Autodesk Inventor part; units mm, degrees
ref_plane "YZ Plane" through (0, 0, 0) normal (1, 0, 0) x (0, 1, 0)
ref_plane "XZ Plane" through (0, 0, 0) normal (0, 1, 0) x (-1, 0, 0)
ref_plane "XY Plane" through (0, 0, 0) normal (0, 0, 1) x (1, 0, 0)
sketch "Szkic1" plane through (0, 0, 0) normal (0, 0, 1) x (1, 0, 0)
  line L0 (6.7664, -3.387) -> (-9.1111, -1.9923)
  arc A0 (6.7664, 3.387) -> (6.7664, -3.387) centre (7.0639, 0) ccw construction
  line L1 (6.7664, 3.387) -> (-9.1111, 1.9923)
  arc A1 (-9.1111, 1.9923) -> (-9.1111, -1.9923) centre (-8.9361, 0) ccw
  circle A2 centre (-5.2361, 0) radius 0.5
  circle A3 centre (-7.1361, 0) radius 0.5
  circle A4 centre (-9.0361, 0) radius 0.5
  circle A5 centre (2.3639, 0) radius 0.5
  circle A6 centre (0.4639, 0) radius 0.5
  circle A7 centre (-1.4361, 0) radius 0.5
  circle A8 centre (-3.3361, 0) radius 0.5
  circle A9 centre (7.0639, 0) radius 3.4 construction
  arc A10 (6.6789, -4.3831) -> (6.6789, 4.3831) centre (7.0639, 0) ccw
  line L2 (6.7664, 3.387) -> (-9.1111, 1.9923)
  line L3 (6.7664, -3.387) -> (-9.1111, -1.9923)
  arc A11 (-9.1111, 1.9923) -> (-9.1111, -1.9923) centre (-8.9361, 0) ccw
  arc A12 (-9.1986, 2.9885) -> (-9.1986, -2.9885) centre (-8.9361, 0) ccw
  line L4 (-9.1986, -2.9885) -> (6.6789, -4.3831)
  line L5 (-9.1986, 2.9885) -> (6.6789, 4.3831)
  circle A13 centre (7.0639, 0) radius 3.4
  line L6 (6.7664, 3.387) -> (-9.1111, 1.9923)
  line L7 (6.7664, -3.387) -> (-9.1111, -1.9923)
  arc A14 (-9.1111, 1.9923) -> (-9.1111, -1.9923) centre (-8.9361, 0) ccw
  dimension "d1" = 1
extrude "Wyciągnięcie proste1" add sketch "Szkic1" along normal blind 2.125 contours L0 A1 L1 A13 | A13 | A2 | A3 | A4 | A5 | A6 | A7 | A8 | L4 A12 L5 A10
sketch "Szkic2" plane through (0, 0, 2.125) normal (0, 0, 1) x (1, 0, 0)
  circle A0 centre (7.0639, 0) radius 3.4
  arc A1 (-9.1111, 1.9923) -> (-9.1111, -1.9923) centre (-8.9361, 0) ccw
  line L0 (6.7664, -3.387) -> (-9.1111, -1.9923)
  line L1 (6.7664, 3.387) -> (-9.1111, 1.9923)
  point P0 (0, 0)
extrude "Wyciągnięcie proste2" cut sketch "Szkic2" against normal blind 2.125
sketch "Szkic3" plane through (0, 0, 0) normal (0, 0, -1) x (-1, 0, 0)
  circle A0 centre (11.4331, 0) radius 0.503
  point P0 (0, 0)
extrude "Wyciągnięcie proste3" add sketch "Szkic3" along normal blind 2.125
properties part number "adapter"
The listing builds one solid part. Answer for the finished solid, in the listing's coordinates (mm). A direction names the side the tool comes from. Coordinates: 2 decimals unless noted, no trailing zeros. Order: outer loops, then holes, each group sorted by start corner. A loop starts at its lowest first (then second) coordinate and runs counter-clockwise, first axis right, second up.
Q1. For a pull along X with two mould halves and no side action, classify faces 1 (the face through (-1.371, -3.676, 1.048)), 2 (the face through (-11.4, 0, -2.125)), 3 (the face through (-1.06, -2.7, 1.08)) as pulls with the +X half, pulls with the -X half, needs draft (parallel to the pull), parting line crosses it, or undercut.
Q2. A cutting plane is placed at A-A, the plane x = 10. Write down the section's boundary in (y, z) (3 decimals).
Q3. A cutting plane is placed at C-C, the plane z = 1.6. Write down the section's boundary in (x, y), and give its area (3 significant figures).
Q4. Consider line 1 (X direction, y = 0, z = 0.7); line 2 (Z direction, x = -2.25, y = -2.75) (3 decimals); line 3 (Y direction, x = -9, z = 0.15). Determine where each line is inside the solid, lowest interval first.
Q5. Given P1, Ø1.5, axis at y = 1, z = -0.5, coming from the +X side; P2, Ø1, axis at y = -2, z = -1, coming from the -X side; P3, Ø2, axis at x = -2, y = -3, coming from the -Z side, each flat-ended and moving along its own axis, determine where each tip first touches the part or whether it passes through.
Q6. A cutting plane is placed at B-B, the plane y = 1.25. Write down the section's boundary in (x, z) (3 decimals), and give its area (3 significant figures).
Q7. A cutting plane is placed at D-D, the plane z = -1.75. Write down the section's boundary in (x, y), and give its area (3 significant figures).
Q8. Which of the six approach directions +Z, -Z, +X, -X, +Y, -Y give full straight-line access (tool end or side, diameter ignored) to faces 4 (the face through (-11.935, -0.062, 1.048)), 5 (the face through (-10.93, -0.02, -1.05)), 6 (the face through (-1.06, 2.7, 1.08))?
Answers follow:
1. face 1: pulls with the -X half
1. face 2: needs draft
1. face 3: undercut
2. outline: (-3.277, 0) - (-1.714, 0) - (-1.714, 2.125) - (-3.277, 2.125) - close; (1.714, 0) - (3.277, 0) - (3.277, 2.125) - (1.714, 2.125) - close
3. outline: (-9.2, -2.99) - (6.68, -4.38) arc R4.4 ccw (long way) to (6.68, 4.38) - (-9.2, 2.99) arc R3 ccw to start; hole (-9.11, -1.99) - (6.77, -3.39) arc R3.4 ccw (long way) to (6.77, 3.39) - (-9.11, 1.99) arc R2 ccw to start
3. area: 52.2 mm2
4. line 1: x = -11.94 to -10.94, 10.46 to 11.46
4. line 2: z = 0 to 2.125
4. line 3: y = -3.01 to -2, 2 to 3.01
5. P1: stops at x = 11.44
5. P2: passes through
5. P3: stops at z = 0
6. outline: (-11.663, 0) - (-10.497, 0) - (-10.497, 2.125) - (-11.663, 2.125) - close; (10.226, 0) - (11.283, 0) - (11.283, 2.125) - (10.226, 2.125) - close
6. area: 4.72 mm2
7. outline: circle Ø1.01 at (-11.43, 0)
7. area: 0.795 mm2
8. face 4: +Z, -Z, -X
8. face 5: -Z
8. face 6: +Z, -Z
